Read the model definition and answer for the solid it produces. Units are mm, in the model's axes. Face numbers are marked on the shaded views. Coordinates: 2 decimals unless noted, no trailing zeros. Write each loop counter-clockwise with the first axis right and the second up, starting at its lowest first coordinate (ties: lowest second). Pieces come first, ordered by that corner, then holes.
1) The part is cut by section A-A (y = 54). Determine the outline of the cut face in (x, z).
2) Find the intervals of material crossed by line 1 (X direction, y = 21, z = 0); line 2 (Z direction, x = -1.5, y = 29.5), in increasing order.
3) Determine the mould class of the marked faces 1 and 2 for opening direction X: +X half, -X half, draft (parallel to the pull), parting line (faces both ways), or undercut.
4) This flat-tipped pin is pushed along its axis until it touches: pin 1 Ø1.5 at (y, z) = (14, 1) entering from +X. Where does it stop, or does it pass through?
from build123d import *

# Parameters (mm, degrees)
SKETCH1_R           = 3.81
BOSS_EXTRUDE1_DEPTH = 67.7
SKETCH5_R           = 0.508
CUT_EXTRUDE2_DEPTH  = 77.390262478
SKETCH7_R           = 2.61
CUT_EXTRUDE3_DEPTH  = 6
CUT_EXTRUDE3_DRAFT  = -19.33
FILLET3_R           = 0.3


with BuildPart() as part:
    # Sketch1 → Boss-Extrude1 (new body)
    with BuildSketch(Plane(origin=(0, 0, 0), x_dir=(1, 0, 0), z_dir=(0, 1, 0))):
        with Locations(Location((0, 0, 0), (0, 0, 270))):
            Circle(SKETCH1_R)
    extrude(amount=BOSS_EXTRUDE1_DEPTH)

    # Loft1: read off the stored shape, not the designer's step
    # Loft1: loft between two sections, ruled curve by curve
    loft1_from = [
        Edge.make_bspline([(1.215970554, 76.2, 1.039911348), (-0.863852142, 76.2, 3.471852456), (-3.29579325, 76.2, 1.39202976), (-1.215970554, 76.2, -1.039911348), (0.863852142, 76.2, -3.471852456), (3.29579325, 76.2, -1.39202976), (1.215970554, 76.2, 1.039911348)], [0, 0, 0, 0, 0.5, 0.5, 0.5, 1, 1, 1, 1], 3, [1, 0.333333333, 0.333333333, 1, 0.333333333, 0.333333333, 1]),
    ]
    loft1_to = [
        Edge.make_bspline([(2.318114705, 67.7, 3.023647501), (-3.729180297, 67.7, 7.659876912), (-8.365409708, 67.7, 1.612581909), (-2.318114705, 67.7, -3.023647501), (3.729180297, 67.7, -7.659876912), (8.365409708, 67.7, -1.612581909), (2.318114705, 67.7, 3.023647501)], [0, 0, 0, 0, 0.5, 0.5, 0.5, 1, 1, 1, 1], 3, [1, 0.333333333, 0.333333333, 1, 0.333333333, 0.333333333, 1]),
    ]
    loft1 = Solid(Shell([*[Face.make_surface_from_curves(loft1_from[k], loft1_to[k]) for k in range(1)], Face(Wire(loft1_from)), Face(Wire(loft1_to))]))
    add(loft1)

    # Sketch5 → Cut-Extrude2 (cut, through all)
    with BuildSketch(Plane(origin=(0, 76.2, 0), x_dir=(1, 0, 0), z_dir=(0, 1, 0))):
        with Locations(Location((0, 0, 0), (0, 0, 270))):
            Circle(SKETCH5_R)
    extrude(amount=-CUT_EXTRUDE2_DEPTH, mode=Mode.SUBTRACT)


with BuildPart() as cut_extrude3_tool:
    # Sketch7 → Cut-Extrude3 (with draft: the straight prism first)
    with BuildSketch(Plane.XZ):
        Circle(SKETCH7_R)
    extrude(amount=-CUT_EXTRUDE3_DEPTH)
    # Cut-Extrude3: the draft: its side faces are tilted about the plane it starts from
    cut_extrude3_sides = [cut_extrude3_tool.faces().sort_by_distance(p)[0] for p in [
        (-2.61, 3, 0),
    ]]
    draft(cut_extrude3_sides, Plane.XZ, CUT_EXTRUDE3_DRAFT)


with BuildPart() as part_1:
    add(part.part)

    # Cut-Extrude3: cut by cut_extrude3_tool
    add(cut_extrude3_tool.part, mode=Mode.SUBTRACT)

    # Fillet3
    fillet3_edges = [part_1.edges().sort_by_distance(p)[0] for p in [
        (0, 0, -3.81),
    ]]
    fillet(fillet3_edges, radius=FILLET3_R)


solid = part_1.part
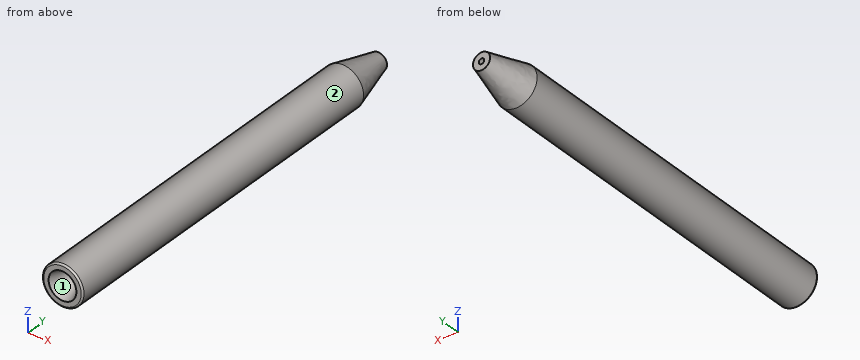
Reported:
1. outline: circle Ø7.62 at (0, 0); hole circle Ø1.02 at (0, 0)
2. line 1: x = -3.81 to -0.51, 0.51 to 3.81
2. line 2: z = -3.5 to 3.5
3. face 1: undercut
3. face 2: parting line
4. pin 1: stops at x = 3.8
